Design review of the part built by this model. Coordinates are the model's own, in mm. A direction names the side the tool comes from. Coordinates: 2 decimals unless noted, no trailing zeros. Write each loop counter-clockwise with the first axis right and the second up, starting at its lowest first coordinate (ties: lowest second). Pieces come first, ordered by that corner, then holes. Notation, with made-up numbers: (83.25, 76.5) - (138.25, 76.5) arc R17 ccw to (138.25, 105.5) - close; hole circle Ø4 at (23.25, -26). An arc over 180 degrees is marked (long way). Answer as a JSON object with one key per item and string values.
```python
from build123d import *

# Parameters (mm, degrees)
BOSS_EXTRUDE1_DEPTH = 2
FILLET1_R           = 1
BOSS_EXTRUDE2_DEPTH = 13.6
SKETCH4_W           = 7
SKETCH4_H           = 11
CUT_EXTRUDE1_DEPTH  = 11.2
SKETCH5_W           = 2
SKETCH5_H           = 11
BOSS_EXTRUDE3_DEPTH = 7
FILLET2_R           = 2
FILLET3_R           = 1


with BuildPart() as part:
    # Sketch1 → Boss-Extrude1 (new body)
    with BuildSketch(Plane.XY):
        Polygon((0, 0), (12, 0), (12, 12), (24, 12), (24, 44.6), (22, 44.6), (22, 50), (5, 50), (5, 52.4), (-10, 52.4), (-10, 50), (-22, 50), (-22, 44.6), (-30, 44.6), (-30, 35.3), (-24, 35.3), (-24, 12), (-12, 12), (-12, 0), align=None)
    extrude(amount=BOSS_EXTRUDE1_DEPTH)

    # Fillet1
    fillet1_edges = [part.edges().sort_by_distance(p)[0] for p in [
        (-12, 0, 1),
        (-12, 12, 1),
        (-24, 12, 1),
        (-30, 35.3, 1),
        (-30, 44.6, 1),
        (-22, 50, 1),
        (-10, 52.4, 1),
        (5, 52.4, 1),
        (22, 50, 1),
        (24, 12, 1),
        (12, 12, 1),
        (12, 0, 1),
    ]]
    fillet(fillet1_edges, radius=FILLET1_R)

    # Sketch3 → Boss-Extrude2 (add)
    with BuildSketch(Plane(origin=(0, 0, 0), x_dir=(-1, 0, 0), z_dir=(0, 0, -1))):
        Polygon((-21.8, 49.7), (-21.8, 14), (-9.8, 14), (-9.8, 2.2), (9.8, 2.2), (9.8, 14), (21.8, 14), (21.8, 49.7), (18, 49.7), (18, 21.8), (-18, 21.8), (-18, 49.7), align=None)
    extrude(amount=BOSS_EXTRUDE2_DEPTH)

    # Sketch4 → Cut-Extrude1 (cut)
    with BuildSketch(Plane.XY.offset(2)):
        with Locations((4.5, 9)):
            Rectangle(SKETCH4_W, SKETCH4_H)
        with Locations((-4.5, 9)):
            Rectangle(SKETCH4_W, SKETCH4_H)
    extrude(amount=-CUT_EXTRUDE1_DEPTH, mode=Mode.SUBTRACT)

    # Sketch5 → Boss-Extrude3 (add)
    with BuildSketch(Plane.XY.offset(2)):
        with Locations((0, 9)):
            Rectangle(SKETCH5_W, SKETCH5_H)
    extrude(amount=BOSS_EXTRUDE3_DEPTH)

    # Fillet2
    fillet2_edges = [part.edges().sort_by_distance(p)[0] for p in [
        (0, 14.5, 9),
        (0, 3.5, 9),
    ]]
    fillet(fillet2_edges, radius=FILLET2_R)

    # Fillet3
    fillet3_edges = [part.edges().sort_by_distance(p)[0] for p in [
        (21.8, 14, -6.8),
        (9.8, 14, -6.8),
        (9.8, 2.2, -6.8),
        (-9.8, 2.2, -6.8),
        (-9.8, 14, -6.8),
        (-21.8, 14, -6.8),
    ]]
    fillet(fillet3_edges, radius=FILLET3_R)


solid = part.part
```
(1) Take a section at C-C, the plane x = -16. Write out the cut boundary in (y, z).
Solved:
{"outline": "(12, 0) - (14, 0) - (14, -13.6) - (21.8, -13.6) - (21.8, 0) - (50, 0) - (50, 2) - (12, 2) - close"}
(2) Take a section at D-D, the plane z = -10. Write out the cut boundary in (x, y).
Solved:
{"outline": "(-21.8, 15) arc R1 ccw to (-20.8, 14) - (-10.8, 14) arc R1 cw to (-9.8, 13) - (-9.8, 3.2) arc R1 ccw to (-8.8, 2.2) - (8.8, 2.2) arc R1 ccw to (9.8, 3.2) - (9.8, 13) arc R1 cw to (10.8, 14) - (20.8, 14) arc R1 ccw to (21.8, 15) - (21.8, 49.7) - (18, 49.7) - (18, 21.8) - (-18, 21.8) - (-18, 49.7) - (-21.8, 49.7) - close"}
(3) Take a section at A-A, the plane z = -3. Write out the cut boundary in (x, y), and give its area (3 significant figures).
Solved:
{"outline": "(-21.8, 15) arc R1 ccw to (-20.8, 14) - (-10.8, 14) arc R1 cw to (-9.8, 13) - (-9.8, 3.2) arc R1 ccw to (-8.8, 2.2) - (8.8, 2.2) arc R1 ccw to (9.8, 3.2) - (9.8, 13) arc R1 cw to (10.8, 14) - (20.8, 14) arc R1 ccw to (21.8, 15) - (21.8, 49.7) - (18, 49.7) - (18, 21.8) - (-18, 21.8) - (-18, 49.7) - (-21.8, 49.7) - close; hole (-8, 3.5) - (-1, 3.5) - (-1, 14.5) - (-8, 14.5) - close; hole (1, 3.5) - (8, 3.5) - (8, 14.5) - (1, 14.5) - close", "area": "629 mm^2"}
(4) Tool access review of faces 1 (the face through (-16, 14, -7)), 2 (the face through (0, 14.5, 4)), 3 (the face through (9.8, 8, -7)), 4 (the face through (-21.8, 32, -7)), 5 (the face through (13, 50, 1)): name each direction out of +Z, -Z, +X, -X, +Y, -Y from which nothing blocks a thin tool from reaching the whole face with its end or side.
Solved:
{"face 1": "-Z, -X, -Y", "face 2": "+Z, +X, -X, +Y", "face 3": "-Z, +X, -Y", "face 4": "-Z, -X, +Y, -Y", "face 5": "+Z, -Z, +X, +Y"}
(5) The part is to be moulded in two halves that separate along Y. For faces 6 (the face through (-24, 24, 1)), 7 (the face through (0, 21.8, -7)), 8 (the face through (-5, 14.5, -4)), say which applies: pulls with the +Y half, pulls with the -Y half, needs draft (parallel to the pull), parting line crosses it, or undercut.
Solved:
{"face 6": "needs draft", "face 7": "pulls with the +Y half", "face 8": "undercut"}
(6) To check wall thickness, follow line 1 (Y direction, x = 2, z = -5.5); line 2 (Y direction, x = -7.5, z = 0.5); line 3 (X direction, y = 39.5, z = -7.75). State the ranges of each line that lie inside material, in increasing order. Write a range as from..to.
Solved:
{"line 1": "y = 2.2..3.5, 14.5..21.8", "line 2": "y = 0..3.5, 14.5..52.4", "line 3": "x = -21.8..-18, 18..21.8"}
(7) For pin 1 (11 mm diameter, centred on x = 1.5, z = -8.5, fed in from -Y); pin 2 (0.6 mm diameter, centred on x = 13, z = 1, fed in from +Y); pin 3 (2 mm diameter, centred on x = 10.5, y = 42, fed in from +Z), all flat-tipped, find the tip position at first contact; note any pin that passes through.
Solved:
{"pin 1": "stops at y = 2.2", "pin 2": "stops at y = 50", "pin 3": "stops at z = 2"}
(8) Take a section at B-B, the plane y = 34. Write out the cut boundary in (x, z), and give its area (3 significant figures).
Solved:
{"outline": "(-24, 0) - (-21.8, 0) - (-21.8, -13.6) - (-18, -13.6) - (-18, 0) - (18, 0) - (18, -13.6) - (21.8, -13.6) - (21.8, 0) - (24, 0) - (24, 2) - (-24, 2) - close", "area": "199 mm^2"}
